```python
from build123d import *

# Parameters (mm, degrees)
ENL_V_MAT_EXTRU_1_DEPTH = 53.396158375


with BuildPart() as part:
    # Esquisse1 → Révolution1 (revolve)
    with BuildSketch(Plane.XY, mode=Mode.PRIVATE) as r_volution1_sk:
        Polygon((-5.08, 36.5125), (5.08, 36.5125), (5.08, 28.8925), (1.905, 28.8925), (1.905, 10.16), (3.81, 10.16), (3.81, 0), (-3.81, 0), (-3.81, 10.16), (-1.905, 10.16), (-1.905, 28.8925), (-5.08, 28.8925), align=None)
    revolve(r_volution1_sk.sketch.rotate(Axis((-12.56603466, 0, 0), (1, 0, 0)), 90), axis=Axis((-12.56603466, 0, 0), (1, 0, 0)))

    # Esquisse2 → Enlèv. mat.-Extru.1 (cut, through all)
    with BuildSketch(Plane(origin=(3.81, 0, 0), x_dir=(0, 0, -1), z_dir=(1, 0, 0))):
        Polygon((0, 7.332348419), (-6.35, 3.666174209), (-6.35, -3.666174209), (0, -7.332348419), (6.35, -3.666174209), (6.35, 3.666174209), align=None)
    extrude(amount=-ENL_V_MAT_EXTRU_1_DEPTH, mode=Mode.SUBTRACT)


solid = part.part
```
For this review, take the finished solid that the model builds, in its own axes (mm). A direction names the side the tool comes from. Coordinates: 2 decimals unless noted, no trailing zeros. Order: outer loops, then holes, each group sorted by start corner. A loop starts at its lowest first (then second) coordinate and runs counter-clockwise, first axis right, second up. Notation, with made-up numbers: (-23, 0) - (13, 0) arc R16 cw to (13, 8) - close; hole circle Ø4 at (26, -36). An arc over 180 degrees is marked (long way). Answer as a JSON object with one key per item and string values. Group by question number.
1. We need section C-C on z = 27.5. State the section outline as (x, y) points (3 decimals).
2. Clearance check with flat-ended pins moving along their axes: P1, Ø3, axis at y = 13.5, z = 7, coming from the +X side (3 decimals); P2, Ø16.5, axis at y = 4.5, z = -5, coming from the -X side; P3, Ø4, axis at x = 0.5, y = -25.5, coming from the -Z side. State where each tip first meets the part, or that it passes through.
3. We need section D-D on y = -19. State the section outline as (x, z) points (3 decimals), then the cut area to 3 significant figures.
4. The part is to be moulded in two halves that separate along Z. For faces 4 (the cylindrical face through (0.07, 32.39, 16.85)), 5 (the flat face through (-1.905, 0, -12)), 6 (the flat face through (5.08, -11, 27)), say which applies: pulls with the +Z half, pulls with the -Z half, needs draft (parallel to the pull), parting line crosses it, or undercut.
5. For probe 1 along Y at (x, z) = (-3.45, 0); probe 2 along Z at (x, y) = (2, -1); probe 3 along Y at (x, z) = (-4.1, 0), list the stretches that pass through material, from the lowest coordinate up.
6. For faces 1 (the cylindrical face through (2.871, -10.074, -1.323)), 2 (the flat face through (0, 0, -6.35)), 3 (the flat face through (-3.81, 0, -7)), list the 3-axis set-ups (+Z, -Z, +X, -X, +Y, -Y) from which the entire face can be reached by the end or side of a thin tool; tool diameter is ignored.
Final values:
{
 "1": {"outline": "(-5.08, -24.019) - (5.08, -24.019) - (5.08, -8.862) - (1.905, -8.862) - (1.905, 8.862) - (5.08, 8.862) - (5.08, 24.019) - (-5.08, 24.019) - (-5.08, 8.862) - (-1.905, 8.862) - (-1.905, -8.862) - (-5.08, -8.862) - close"},
 "2": {"P1": "x = 1.905", "P2": "x = -3.81", "P3": "z = -27.94"},
 "3": {"outline": "(-5.08, -31.18) - (5.08, -31.18) - (5.08, -21.766) - (1.905, -21.766) - (1.905, 21.766) - (5.08, 21.766) - (5.08, 31.18) - (-5.08, 31.18) - (-5.08, 21.766) - (-1.905, 21.766) - (-1.905, -21.766) - (-5.08, -21.766) - close", "area": "357 mm²"},
 "4": {"face 4": "parting line crosses it", "face 5": "undercut", "face 6": "needs draft"},
 "5": {"probe 1": "-36.51 to -28.89, -10.16 to -7.33, 7.33 to 10.16, 28.89 to 36.51", "probe 2": "-36.5 to -28.88, -10.11 to -6.35, 6.35 to 10.11, 28.88 to 36.5", "probe 3": "-36.51 to -28.89, 28.89 to 36.51"},
 "6": {"face 1": "+X", "face 2": "+X, -X", "face 3": "-X"}
}
